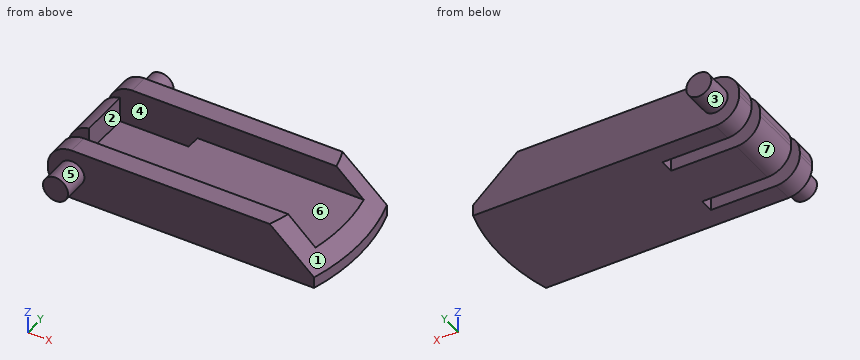
```python
from build123d import *

# Parameters (mm, degrees)
F1_DEPTH     = 2.45
F2_W         = 1.91
F2_H         = 1.91
F2_H_2       = 4.81
F3_DEPTH     = 2.38
F4_T1_DEPTH  = 13.3148286025
F4_T3_DEPTH  = 7.6124143012
F4_T5_DEPTH  = 13.3148286025
F4_T7_DEPTH  = 16.0629874681
F4_T9_DEPTH  = 16.2148286025
F4_T14_DEPTH = 13.3148286025
F5_T2_ANGLE  = 64.9142912697
F5_T4_ANGLE  = 64.9142912697
F6_R         = 1.19
F7_DEPTH     = 2.54


# Not quite as in the source:
# - a fillet or chamfer that OpenCascade refuses, or shapes differently, is made with other operations: its cross-section is extruded or revolved along the edge and cut away or added


with BuildPart() as f1:
    # F0 (on Top) → F1 (new body)
    with BuildSketch(Plane.XY):
        Polygon((12.22, -5.655), (12.22, 5.655), (-7.02, 5.655), (-9.51, 5.655), (-13.04, 5.655), (-13.04, 3.745), (-4.6004378237, 3.745), (-4.6004378237, 2.405), (-13.04, 2.405), (-13.04, -2.405), (-4.6004378237, -2.405), (-4.6004378237, -3.745), (-13.04, -3.745), (-13.04, -5.655), (-9.51, -5.655), (-7.02, -5.655), align=None)
        with BuildLine():
            ThreePointArc((12.22, -5.655), (13.04, 0), (12.22, 5.655))
            Line((12.22, 5.655), (12.22, -5.655))
        make_face()
    extrude(amount=F1_DEPTH)

    # F2 (on face) → F3 (join)
    with BuildSketch(Plane.XY.offset(2.45)):
        with BuildLine():
            ThreePointArc((12.6846069362, 3.745), (12.4758901154, 4.705737445), (12.22, 5.655))
            Line((12.22, 5.655), (-11.13, 5.655))
            Line((-11.13, 5.655), (-11.13, 3.745))
            Line((-11.13, 3.745), (-4.6004378237, 3.745))
            Line((-4.6004378237, 3.745), (12.6846069362, 3.745))
        make_face()
        with Locations((-12.085, 4.7)):
            Rectangle(F2_W, F2_H)
        with Locations((-12.085, 0)):
            Rectangle(F2_W, F2_H_2)
        with Locations((-12.085, -4.7)):
            Rectangle(F2_W, F2_H)
        with BuildLine():
            ThreePointArc((12.22, -5.655), (12.4758901154, -4.705737445), (12.6846069362, -3.745))
            Line((12.6846069362, -3.745), (-4.6004378237, -3.745))
            Line((-4.6004378237, -3.745), (-11.13, -3.745))
            Line((-11.13, -3.745), (-11.13, -5.655))
            Line((-11.13, -5.655), (12.22, -5.655))
        make_face()
    extrude(amount=F3_DEPTH)

    # F4: fillet of radius 2.28 on 6 edges, made by hand

    # F4_s2 → F4_t1 (cut)
    with BuildSketch(Plane.XZ.offset(-1.9574143012)):
        with BuildLine():
            ThreePointArc((-10.7590343146, -0.0004), (-12.3722034611, 0.6677965389), (-13.0404, 2.2809656854))
            Line((-13.0404, 2.2809656854), (-13.2685365685, 2.2809656854))
            ThreePointArc((-13.2685365685, 2.2809656854), (-13.2681365685, 1.1404828427), (-13.2681365685, 0))
            Line((-13.2681365685, 0), (-13.04, -0.2281365685))
            ThreePointArc((-13.04, -0.2281365685), (-11.8995171573, -0.2281365685), (-10.7590343146, -0.2285365685))
            Line((-10.7590343146, -0.2285365685), (-10.7590343146, -0.0004))
        make_face()
    extrude(amount=F4_T1_DEPTH, mode=Mode.SUBTRACT)

    # F4_s4 → F4_t3 (cut)
    with BuildSketch(Plane.XZ.offset(-11.3574143012)):
        with BuildLine():
            ThreePointArc((-10.7590343146, 4.8304), (-12.3722034611, 4.1622034611), (-13.0404, 2.5490343146))
            Line((-13.0404, 2.5490343146), (-13.2685365685, 2.5490343146))
            ThreePointArc((-13.2685365685, 2.5490343146), (-13.2681365685, 3.6895171573), (-13.2681365685, 4.83))
            Line((-13.2681365685, 4.83), (-13.04, 5.0581365685))
            ThreePointArc((-13.04, 5.0581365685), (-11.8995171573, 5.0581365685), (-10.7590343146, 5.0585365685))
            Line((-10.7590343146, 5.0585365685), (-10.7590343146, 4.8304))
        make_face()
    extrude(amount=F4_T3_DEPTH, mode=Mode.SUBTRACT)

    # F4_s6 → F4_t5 (cut)
    with BuildSketch(Plane.XZ.offset(-11.3574143012)):
        with BuildLine():
            ThreePointArc((-10.7590343146, -0.0004), (-12.3722034611, 0.6677965389), (-13.0404, 2.2809656854))
            Line((-13.0404, 2.2809656854), (-13.2685365685, 2.2809656854))
            ThreePointArc((-13.2685365685, 2.2809656854), (-13.2681365685, 1.1404828427), (-13.2681365685, 0))
            Line((-13.2681365685, 0), (-13.04, -0.2281365685))
            ThreePointArc((-13.04, -0.2281365685), (-11.8995171573, -0.2281365685), (-10.7590343146, -0.2285365685))
            Line((-10.7590343146, -0.2285365685), (-10.7590343146, -0.0004))
        make_face()
    extrude(amount=F4_T5_DEPTH, mode=Mode.SUBTRACT)

    # F4_s8 → F4_t7 (cut)
    with BuildSketch(Plane.XZ.offset(-8.0314937341)):
        with BuildLine():
            ThreePointArc((-11.1300650541, 4.8303946745), (-12.4984431492, 4.0555753965), (-13.0404, 2.5794025419))
            Line((-13.0404, 2.5794025419), (-13.2685365685, 2.5794025419))
            ThreePointArc((-13.2685365685, 2.5794025419), (-13.2681365685, 3.704701271), (-13.2681365685, 4.83))
            Line((-13.2681365685, 4.83), (-13.04, 5.0581365685))
            ThreePointArc((-13.04, 5.0581365685), (-12.0850325271, 5.0581365685), (-11.1671681281, 5.0554938878))
            Line((-11.1671681281, 5.0554938878), (-11.1300650541, 4.8303946745))
        make_face()
    extrude(amount=F4_T7_DEPTH, mode=Mode.SUBTRACT)

    # F4_s10 → F4_t9 (cut)
    with BuildSketch(Plane.XZ.offset(-8.1074143012)):
        with BuildLine():
            ThreePointArc((-10.7590343146, -0.0004), (-12.3722034611, 0.6677965389), (-13.0404, 2.2809656854))
            Line((-13.0404, 2.2809656854), (-13.2685365685, 2.2809656854))
            ThreePointArc((-13.2685365685, 2.2809656854), (-13.2681365685, 1.1404828427), (-13.2681365685, 0))
            Line((-13.2681365685, 0), (-13.04, -0.2281365685))
            ThreePointArc((-13.04, -0.2281365685), (-11.8995171573, -0.2281365685), (-10.7590343146, -0.2285365685))
            Line((-10.7590343146, -0.2285365685), (-10.7590343146, -0.0004))
        make_face()
    extrude(amount=F4_T9_DEPTH, mode=Mode.SUBTRACT)


with BuildPart() as f4_tool12:
    # F4_s13 → F4_t14 (new body)
    with BuildSketch(Plane.XZ.offset(-1.9574143012)):
        with BuildLine():
            ThreePointArc((-10.7590343146, 4.8304), (-12.3722034611, 4.1622034611), (-13.0404, 2.5490343146))
            Line((-13.0404, 2.5490343146), (-13.2685365685, 2.5490343146))
            ThreePointArc((-13.2685365685, 2.5490343146), (-13.2681365685, 3.6895171573), (-13.2681365685, 4.83))
            Line((-13.2681365685, 4.83), (-13.04, 5.0581365685))
            ThreePointArc((-13.04, 5.0581365685), (-11.8995171573, 5.0581365685), (-10.7590343146, 5.0585365685))
            Line((-10.7590343146, 5.0585365685), (-10.7590343146, 4.8304))
        make_face()
    extrude(amount=F4_T14_DEPTH)

    split(bisect_by=Plane.XZ.offset(2.405), keep=Keep.TOP)


with BuildPart() as f1_1:
    add(f1.part)

    # F4_t11: cut F4_tool12
    add(f4_tool12.part, mode=Mode.SUBTRACT)

    # F5: chamfer of 4 x 3.76 on 2 edges, made by hand

    # F5_s1 → F5_t2 (revolve, cut)
    with BuildSketch(Plane(origin=(-0.7123621612, -2.0942885882, 0), x_dir=(0, 0, 1), z_dir=(-0.3220259314, -0.9467308485, 0))):
        Polygon((4.83, -9.4059274017), (1.07, -13.4059274017), (4.83, -13.4059274017), align=None)
    revolve(axis=Axis((-6.8694054878, 0, 4.83), (0, 0, 1)), revolution_arc=F5_T2_ANGLE, mode=Mode.SUBTRACT)

    # F5_s3 → F5_t4 (revolve, cut)
    with BuildSketch(Plane(origin=(-3.5700040609, -3.4320367849, 0), x_dir=(0, 0, 1), z_dir=(-0.7208995903, -0.6930395232, 0))):
        Polygon((4.83, -11.148635984), (1.07, -15.148635984), (4.83, -15.148635984), align=None)
    revolve(axis=Axis((-6.8694054878, 0, 4.83), (0, 0, 1)), revolution_arc=F5_T4_ANGLE, mode=Mode.SUBTRACT)

    # F6 (on face) → F7 (join)
    with BuildSketch(Plane.XZ.offset(5.655)):
        with Locations((-10.76, 2.55)):
            Circle(F6_R)
    extrude(amount=F7_DEPTH)

    # F8: F1 across plane


with BuildPart() as f1_2:
    add(f1_1.part)
    add(f1_1.part.mirror(Plane.XZ))


solid = f1_2.part
```
The model under review builds one solid part; all positions refer to its coordinate system, in mm. Face numbers are marked on the shaded views. A direction names the side the tool comes from. Coordinates: 2 decimals unless noted, no trailing zeros. Order: outer loops, then holes, each group sorted by start corner. A loop starts at its lowest first (then second) coordinate and runs counter-clockwise, first axis right, second up. Notation, with made-up numbers: (24.5, -23.5) -> (71.5, -23.5) arc R31 cw to (71.5, 5.5) -> close; hole circle Ø5 at (-32, 51). An arc over 180 degrees is marked (long way). Answer in a Markdown table with one row per item. Add a question column.
Item 1: We need section A-A on x = 0.25. Write out the cut boundary in (y, z) (3 decimals).
Item 2: To check wall thickness, follow probe 1 along Y at (x, z) = (-1.75, 4) (3 decimals); probe 2 along Y at (x, z) = (-1.25, 1.1) (3 decimals); probe 3 along Z at (x, y) = (-3.5, 3). State the ranges of each line that lie inside material, in increasing order.
Item 3: We need section C-C on y = 6.25. Write out the cut boundary in (x, z), plus the area to 3 significant figures.
Item 4: Machinability: for the marked faces 4, 5, 6 and 7, which of the approach directions +Z, -Z, +X, -X, +Y, -Y give a long, thin tool a straight path to every point of the face, cutting with its end or side? Answer none if there is none.
Item 5: Mouldability with a two-part tool opening along Y and no side actions: class the marked faces 1, 2 and 3 as +Y half, -Y half, draft (parallel to the pull), parting line (faces both ways), or undercut.
Item 6: We need section B-B on z = 3. Write out the cut boundary in (x, y) (3 decimals).
Item 7: Clearance check with flat-ended pins moving along their axes: pin 1 (3.5 mm diameter, centred on x = -5, y = 1.5, fed in from +Z); pin 2 (2.5 mm diameter, centred on y = -0.5, z = 3, fed in from +X); pin 3 (1.4 mm diameter, centred on x = -8, z = 3, fed in from +Y) (3 decimals); pin 4 (5 mm diameter, centred on x = -8, y = 6.5, fed in from -Z). State where each tip first meets the part, or that it passes through.
Final values:
| question | item | result |
|---|---|---|
| 1 | outline | (-5.655, 0) -> (5.655, 0) -> (5.655, 4.83) -> (3.745, 4.83) -> (3.745, 2.45) -> (-3.745, 2.45) -> (-3.745, 4.83) -> (-5.655, 4.83) -> close |
| 2 | probe 1 | y = -5.655 to -3.745, 3.745 to 5.655 |
| 2 | probe 2 | y = -5.655 to 5.655 |
| 2 | probe 3 | z = 0 to 2.45 |
| 3 | outline | circle Ø2.38 at (-10.76, 2.55) |
| 3 | area | 4.45 mm2 |
| 4 | face 4 | +Z, -X |
| 4 | face 5 | -Y |
| 4 | face 6 | +Z, +X |
| 4 | face 7 | -Z, -X, +Y, -Y |
| 5 | face 1 | parting line |
| 5 | face 2 | undercut |
| 5 | face 3 | draft |
| 6 | outline | (-13.001, -2.405) -> (-11.13, -2.405) -> (-11.13, 2.405) -> (-13.001, 2.405) -> close; (-12.995, -5.655) -> (-11.862, -5.655) -> (-11.862, -8.195) -> (-9.658, -8.195) -> (-9.658, -5.655) -> (10.068, -5.655) arc R17.856 ccw to (10.59, -3.745) -> (-12.995, -3.745) -> close; (-12.995, 3.745) -> (10.59, 3.745) arc R17.856 ccw to (10.068, 5.655) -> (-9.658, 5.655) -> (-9.658, 8.195) -> (-11.862, 8.195) -> (-11.862, 5.655) -> (-12.995, 5.655) -> close |
| 7 | pin 1 | stops at z = 2.45 |
| 7 | pin 2 | stops at x = 12.31 |
| 7 | pin 3 | stops at y = 5.655 |
| 7 | pin 4 | stops at z = 0 |
